```python
from build123d import *

# Parameters (mm, degrees)
F0_R     = 70
F0_R_2   = 50
F1_DEPTH = 15
F3_R     = 57.5
F3_R_2   = 50
F4_DEPTH = 3
F5_R     = 57.5
F5_R_2   = 50
F6_DEPTH = 3


with BuildPart() as f1:
    # F0 (on Top) → F1 (new body)
    with BuildSketch(Plane.XY):
        Circle(F0_R)
        Circle(F0_R_2, mode=Mode.SUBTRACT)
    extrude(amount=F1_DEPTH)

    # F3 (on face) → F4 (join)
    with BuildSketch(Plane.XY.offset(15)):
        Circle(F3_R)
        Circle(F3_R_2, mode=Mode.SUBTRACT)
    extrude(amount=F4_DEPTH)

    # F5 (on face) → F6 (cut)
    with BuildSketch(Plane(origin=(0, 0, 0), x_dir=(1, 0, 0), z_dir=(0, 0, -1))):
        Circle(F5_R)
        Circle(F5_R_2, mode=Mode.SUBTRACT)
    extrude(amount=-F6_DEPTH, mode=Mode.SUBTRACT)


solid = f1.part
```
Input: part model. Units: mm. Frame: model coordinates. A direction names the side the tool comes from. Give positions to 0.01 mm unless a question says otherwise; leave off trailing zeros. Order: outer loops, then holes, each group sorted by start corner. A loop starts at its lowest first (then second) coordinate and runs counter-clockwise, first axis right, second up. Notation, with made-up numbers: (44, -11) -> (82, -11) arc R22 cw to (82, 21) -> close; hole circle Ø3 at (8.5, -28.75). An arc over 180 degrees is marked (long way). Write each question's results on one line, items separated by ' | '. Start each with the question number.
Item 1: Contact query for flat-ended pins moving along their axis: P1, Ø3, axis at y = -41.5, z = 13, coming from the -X side; P2, Ø6, axis at x = 48, z = 9.5, coming from the +Y side; P3, Ø1.5, axis at y = 19.5, z = 13.5, coming from the +X side; P4, Ø8, axis at x = -6.5, y = 41.5, coming from the -Z side. Output: stop coordinate, or through.
Item 2: Mould query, pull axis Y, two halves, no side actions, for faces 4 (the cylindrical face through (-12.465, -56.133, 16.479)), 5 (the flat face through (-17.3, -47.1, 3)), 6 (the flat face through (-5.5, 57.4, 0)). Classes: pulls with the +Y half, pulls with the -Y half, needs draft (parallel to the pull), parting line crosses it, or undercut.
Item 3: Cut plane B-B on y = -40. Return the cut outline in (x, z).
Item 4: Cut plane C-C on z = 7.5. Return the cut outline in (x, y), then the cut area to 3 significant figures.
Item 5: Cut plane A-A on x = 0. Return the cut outline in (y, z).
Item 6: Set-up query: faces 1 (the flat face through (-5.5, 57.4, 15)), 2 (the cylindrical face through (47.69, 15.02, 10.4)), 3 (the cylindrical face through (-12.465, 56.133, 1.479)). Return all of +Z, -Z, +X, -X, +Y, -Y with unobstructed straight access to the full face (end or side cutting, diameter ignored); none if empty.
Item 7: Line query: line 1 (Y direction, x = 0, z = 13.5); line 2 (Y direction, x = 0, z = 0.9); line 3 (Z direction, x = 60, y = -26.5). Output: solid intervals per line, ascending.
Item 8: Cut plane D-D on x = -53.5. Return the cut outline in (y, z), then the cut area to 3 significant figures.
Established:
1) P1: x = -57.45 | P2: y = 53.62 | P3: x = 67.44 | P4: through
2) face 4: parting line crosses it | face 5: undercut | face 6: needs draft
3) outline: (-57.45, 0) -> (-41.31, 0) -> (-41.31, 3) -> (-30, 3) -> (-30, 18) -> (-41.31, 18) -> (-41.31, 15) -> (-57.45, 15) -> close; (30, 3) -> (41.31, 3) -> (41.31, 0) -> (57.45, 0) -> (57.45, 15) -> (41.31, 15) -> (41.31, 18) -> (30, 18) -> close
4) outline: circle Ø140 at (0, 0); hole circle Ø100 at (0, 0) | area: 7,540 mm^2
5) outline: (-70, 0) -> (-57.5, 0) -> (-57.5, 3) -> (-50, 3) -> (-50, 18) -> (-57.5, 18) -> (-57.5, 15) -> (-70, 15) -> close; (50, 3) -> (57.5, 3) -> (57.5, 0) -> (70, 0) -> (70, 15) -> (57.5, 15) -> (57.5, 18) -> (50, 18) -> close
6) face 1: +Z | face 2: +Z, -Z | face 3: -Z
7) line 1: -70 to -50, 50 to 70 | line 2: -70 to -57.5, 57.5 to 70 | line 3: 0 to 15
8) outline: (-45.14, 0) -> (-21.07, 0) -> (-21.07, 3) -> (21.07, 3) -> (21.07, 0) -> (45.14, 0) -> (45.14, 15) -> (21.07, 15) -> (21.07, 18) -> (-21.07, 18) -> (-21.07, 15) -> (-45.14, 15) -> close | area: 1,350 mm^2
